Geometry: final body of the model. Coordinates: model frame, mm. A direction names the side the tool comes from. Round coordinates to 2 decimals unless told otherwise and drop trailing zeros. Write each loop counter-clockwise with the first axis right and the second up, starting at its lowest first coordinate (ties: lowest second). Pieces come first, ordered by that corner, then holes. Notation, with made-up numbers: M 15,5.5 L 34,5.5 A16 cw 34,28.5 Z; hole C -35.5,86.5 d10. An arc over 180 degrees is marked long. Use one line per item in the form item = value. Start each with the question number.
Item 1: Ray query, probe 1 along Y at (x, z) = (0, -0.55); probe 2 along Y at (x, z) = (1, 4); probe 3 along Z at (x, y) = (-8.25, 19). Return the intervals inside material, ascending.
Item 2: Section query A-A (y = -18). Return loops of the section in (x, z), and give its area (3 significant figures).
Item 3: Section query C-C (x = 0). Return loops of the section in (y, z).
Item 4: Pull-direction query (Y, two-part tool) for faces 1 (the cylindrical face through (-0.26, 16.83, -0.99)), 2 (the flat face through (-2.5, 21, -1)), 3 (the flat face through (0, 21.75, -1)); classes: pulls with the +Y half, pulls with the -Y half, needs draft (parallel to the pull), parting line crosses it, or undercut.
Item 5: Reachability of faces 4 (the flat face through (2.5, 21, -1)), 5 (the flat face through (8.5, 0, -1)), 6 (the flat face through (-9, 0, 0)), 7 (the flat face through (2.5, -21, -1)) from +Z, -Z, +X, -X, +Y, -Y: full face, straight path, thin tool, end or side. Return the list, or none.
Item 6: Section query B-B (z = -0.75). Return loops of the section in (x, y), and give its area (3 significant figures).
Item 7: Section query D-D (y = -6). Return loops of the section in (x, z), and give its area (3 significant figures).
Item 8: Pin query (flat end, axial travel): pin 1 Ø1.1 at (y, z) = (-21, -0.5) entering from +X; pin 2 Ø0.6 at (x, z) = (-6.5, -1) entering from -Y; pin 3 Ø1.1 at (y, z) = (21, -1) entering from -X. Return the tip coordinate at first contact, or that it passes through.
from build123d import *

# Parameters (mm, degrees)
SKETCH1_W                = 20
SKETCH1_H                = 31.3
BOSS_EXTRUDE1_DEPTH      = 6
SKETCH2_W                = 17
SKETCH2_H                = 41.5
BOSS_EXTRUDE2_DEPTH      = 2
SKETCH3_W                = 5
SKETCH3_H                = 43.5
BOSS_EXTRUDE3_DEPTH      = 2
M2_CLEARANCE_HOLE1_D     = 2.4
M2_CLEARANCE_HOLE1_DEPTH = 2


with BuildPart() as part:
    # Sketch1 → Boss-Extrude1 (new body)
    with BuildSketch(Plane.XY):
        Rectangle(SKETCH1_W, SKETCH1_H)
    extrude(amount=BOSS_EXTRUDE1_DEPTH)

    # Sketch2 → Boss-Extrude2 (add)
    with BuildSketch(Plane(origin=(0, 0, 0), x_dir=(-1, 0, 0), z_dir=(0, 0, -1))):
        Rectangle(SKETCH2_W, SKETCH2_H)
    extrude(amount=BOSS_EXTRUDE2_DEPTH)

    # Sketch3 → Boss-Extrude3 (add)
    with BuildSketch(Plane(origin=(0, 0, -2), x_dir=(-1, 0, 0), z_dir=(0, 0, -1))):
        Rectangle(SKETCH3_W, SKETCH3_H)
    extrude(amount=-BOSS_EXTRUDE3_DEPTH)

    # M2 Clearance Hole1
    with Locations(Plane(origin=(0, 0, -2), x_dir=(-1, 0, 0), z_dir=(0, 0, -1))):
        with Locations((0, 18), (0, -18)):
            Hole(M2_CLEARANCE_HOLE1_D / 2, depth=M2_CLEARANCE_HOLE1_DEPTH)


solid = part.part
Working result:
q1.probe_1 = -21.75 to -19.2, -16.8 to 16.8, 19.2 to 21.75
q1.probe_2 = -15.65 to 15.65
q1.probe_3 = -2 to 0
q2.outline = M -8.5,-2 L -1.2,-2 L -1.2,0 L -8.5,0 Z; M 1.2,-2 L 8.5,-2 L 8.5,0 L 1.2,0 Z
q2.area = 29.2 mm²
q3.outline = M -21.75,-2 L -19.2,-2 L -19.2,0 L -21.75,0 Z; M -16.8,-2 L 16.8,-2 L 16.8,0 L 15.65,0 L 15.65,6 L -15.65,6 L -15.65,0 L -16.8,0 Z; M 19.2,-2 L 21.75,-2 L 21.75,0 L 19.2,0 Z
q4.face_1 = undercut
q4.face_2 = needs draft
q4.face_3 = pulls with the +Y half
q5.face_4 = +Z, -Z, +X, +Y
q5.face_5 = -Z, +X, +Y, -Y
q5.face_6 = -Z, -X, +Y, -Y
q5.face_7 = +Z, -Z, +X, -Y
q6.outline = M -8.5,-20.75 L -2.5,-20.75 L -2.5,-21.75 L 2.5,-21.75 L 2.5,-20.75 L 8.5,-20.75 L 8.5,20.75 L 2.5,20.75 L 2.5,21.75 L -2.5,21.75 L -2.5,20.75 L -8.5,20.75 Z; hole C 0,-18 d2.4; hole C 0,18 d2.4
q6.area = 706 mm²
q7.outline = M -10,0 L -8.5,0 L -8.5,-2 L 8.5,-2 L 8.5,0 L 10,0 L 10,6 L -10,6 Z
q7.area = 154 mm²
q8.pin_1 = 8.5
q8.pin_2 = -20.75
q8.pin_3 = -8.5
